from build123d import *

# Parameters (mm, degrees)
EXTRUDE_1_DEPTH              = 10
SKETCH_2_R                   = 11
CUT_EXTRUDE_1_DEPTH          = 87.058119896
HOLE_WIZARD_M4_1_D           = 4.5
HOLE_WIZARD_M4_1_CBORE_D     = 8
HOLE_WIZARD_M4_1_CBORE_DEPTH = 4.6
SKETCH_3_R                   = 1.2295
CUT_EXTRUDE_2_DEPTH          = 87.058119896


with BuildPart() as part:
    # 草图1 → 凸台-拉伸1 (new body)
    with BuildSketch(Plane.XY):
        Polygon((0, 0), (75, 0), (75, 15), (60, 15), (60, 41), (15, 41), (15, 15), (0, 15), align=None)
    extrude(amount=EXTRUDE_1_DEPTH)

    # 草图2 → 切除-拉伸1 (cut, through all)
    with BuildSketch(Plane.XY.offset(10)):
        with Locations((37.5, 20)):
            Circle(SKETCH_2_R)
    extrude(amount=-CUT_EXTRUDE_1_DEPTH, mode=Mode.SUBTRACT)

    # M4 六角圆柱头螺钉的柱形沉头孔1 (through all)
    with Locations(Plane(origin=(8, 15, 5), x_dir=(1, 0, 0), z_dir=(0, 1, 0))):
        with Locations((0, 0), (59, 0)):
            CounterBoreHole(HOLE_WIZARD_M4_1_D / 2, HOLE_WIZARD_M4_1_CBORE_D / 2, HOLE_WIZARD_M4_1_CBORE_DEPTH)

    # 草图3 → 切除-拉伸2 (cut, through all)
    with BuildSketch(Plane(origin=(0, 0, 0), x_dir=(-1, 0, 0), z_dir=(0, 0, -1))):
        with Locations((-22, 4.5)):
            Circle(SKETCH_3_R)
        with Locations(Location((-53, 4.5, 0), (0, 0, 180))):
            Circle(SKETCH_3_R)
        with Locations((-53, 35.5)):
            Circle(SKETCH_3_R)
        with Locations(Location((-22, 35.5, 0), (0, 0, 180))):
            Circle(SKETCH_3_R)
    extrude(amount=-CUT_EXTRUDE_2_DEPTH, mode=Mode.SUBTRACT)


solid = part.part
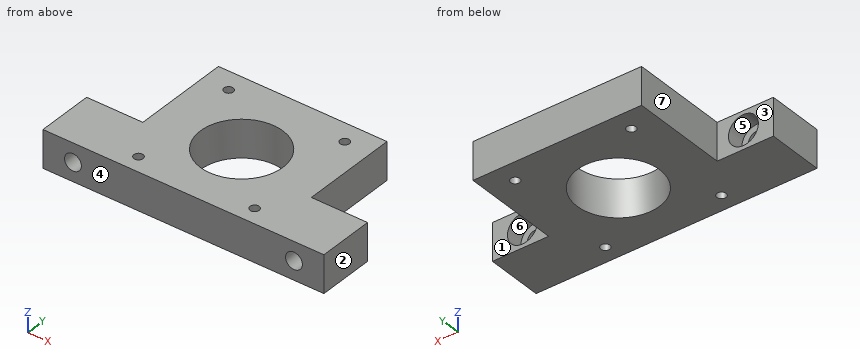
Source: CAD feature listing. Evaluate the final solid. Frame: model axes, mm. Face numbers are marked on the shaded views. A direction names the side the tool comes from. Coordinates: 2 decimals unless noted, no trailing zeros. Loops run counter-clockwise (first coordinate to the right, second up) from the corner with the lowest first, then second, coordinate; pieces in that order, holes last. Notation, with made-up numbers: (69, 22.25) - (84, 22.25) arc R26 ccw to (84, 57.25) - close; hole circle Ø8 at (5, 87.25). An arc over 180 degrees is marked (long way). One line per item, written item: value. Start each with the question number.
1. Section D-D (y = 13). Return the cut outline in (x, z), and give its area (3 significant figures).
2. Ray query, L1, parallel to Y at x = 22, z = 2.75; L2, parallel to X at y = 2, z = 6.5; L3, parallel to X at y = 12.5, z = 6.5. Return the intervals inside material, ascending.
3. Section B-B (y = 35.5). Return the cut outline in (x, z), and give its area (3 significant figures).
4. Set-up query: the marked faces 1, 2 and 3. Return all of +Z, -Z, +X, -X, +Y, -Y with unobstructed straight access to the full face (end or side cutting, diameter ignored); none if empty.
5. Mould query, pull axis X, two halves, no side actions, for the marked faces 4, 5, 6 and 7. Classes: pulls with the +X half, pulls with the -X half, needs draft (parallel to the pull), parting line crosses it, or undercut.
6. Section C-C (x = 8). Return the cut outline in (y, z), and give its area (3 significant figures).
7. Contact query for flat-ended pins moving along their axis: P1, Ø5, axis at x = 67, z = 5, coming from the +Y side; P2, Ø5, axis at x = 69, z = 5, coming from the +Y side; P3, Ø6, axis at y = 34.5, z = 2.5, coming from the +X side. Output: stop coordinate, or through.
8. Section A-A (z = 5). State how many separate pieces and enclosed holes the cut face has, and give its area (3 significant figures).
Verdict:
1. outline: (0, 0) - (29.01, 0) - (29.01, 10) - (0, 10) - close; (45.99, 0) - (75, 0) - (75, 10) - (45.99, 10) - close; hole circle Ø8 at (8, 5); hole circle Ø8 at (67, 5)
1. area: 480 mm2
2. L1: y = 0 to 3.27, 5.73 to 34.27, 36.73 to 41
2. L2: x = 0 to 6.32, 9.68 to 65.32, 68.68 to 75
2. L3: x = 0 to 4.29, 11.71 to 29.45, 45.55 to 63.29, 70.71 to 75
3. outline: (15, 0) - (20.77, 0) - (20.77, 10) - (15, 10) - close; (23.23, 0) - (51.77, 0) - (51.77, 10) - (23.23, 10) - close; (54.23, 0) - (60, 0) - (60, 10) - (54.23, 10) - close
3. area: 401 mm2
4. face 1: +Z, -Z, +X, +Y
4. face 2: +Z, -Z, +X, +Y, -Y
4. face 3: +Z, -Z, -X, +Y
5. face 4: needs draft
5. face 5: undercut
5. face 6: undercut
5. face 7: pulls with the -X half
6. outline: (0, 0) - (15, 0) - (15, 1) - (10.4, 1) - (10.4, 2.75) - (0, 2.75) - close; (0, 7.25) - (10.4, 7.25) - (10.4, 9) - (15, 9) - (15, 10) - (0, 10) - close
6. area: 66.4 mm2
7. P1: stops at y = 10.4
7. P2: stops at y = 15
7. P3: stops at x = 60
8. separate pieces: 3
8. enclosed holes: 5
8. area: 1,730 mm2
